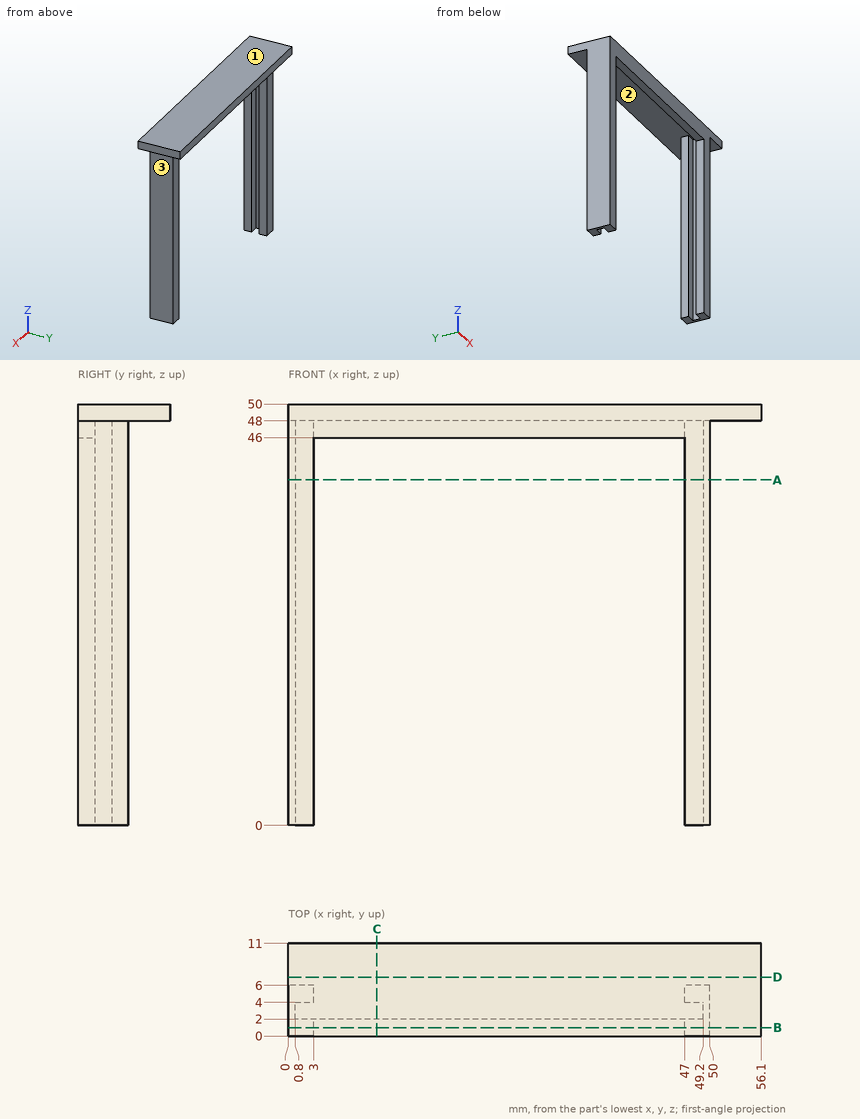
Design review of the part shown in the three views and the two pictorial views. Dimensions are in mm from the part's minimum x, y and z. Round coordinates to 2 decimals unless told otherwise and drop trailing zeros. Loops run counter-clockwise (first coordinate to the right, second up) from the corner with the lowest first, then second, coordinate; pieces in that order, holes last. Notation, with made-up numbers: (60.25, -15) -> (81.25, -15) arc R20 ccw to (81.25, -8) -> close; hole circle Ø10 at (-5.75, -15.75). An arc over 180 degrees is marked (long way). Use one line per item in the form item = value. Start each with the question number.
Q1. We need section D-D on y = 7. Give the boundary of the cut face in (x, z), then the cut area to 3 significant figures.
Q2. We need section B-B on y = 1. Give the boundary of the cut face in (x, z).
Q3. We need section C-C on x = 10.5. Give the boundary of the cut face in (y, z), then the cut area to 3 significant figures.
Q4. We need section A-A on z = 41. Give the boundary of the cut face in (x, y), then the cut area to 3 significant figures.
Q5. Wall thickness on line 1 along X through (y, z) = (5.75, 16); line 2 along X through (y, z) = (3.75, 39); line 3 along Z through (x, y) = (30, 10.25): over which ranges is each line inside the solid? List them lowest first. Write a range as [from, to].
Q6. For pin 1 Ø1 at (y, z) = (4.5, 23.5) entering from -X; pin 2 Ø14.5 at (x, z) = (14, 25.5) entering from +Y; pin 3 Ø0.9 at (x, z) = (48.5, 19) entering from +Y; pin 4 Ø2 at (x, y) = (39, 7) entering from -Z, all flat-tipped, find the tip position at first contact; note any pin that passes through.
Q7. Draft analysis for pull direction X (two halves, no side actions). For the marked faces 1, 2 and 3, state which applies: +X half, -X half, draft (parallel to the pull), parting line (faces both ways), or undercut.
Calculated:
q1.outline = (0, 48) -> (56.1, 48) -> (56.1, 50) -> (0, 50) -> close
q1.area = 112 mm²
q2.outline = (0, 0) -> (3, 0) -> (3, 46) -> (47, 46) -> (47, 0) -> (50, 0) -> (50, 48) -> (56.1, 48) -> (56.1, 50) -> (0, 50) -> close
q3.outline = (0, 46) -> (2, 46) -> (2, 48) -> (11, 48) -> (11, 50) -> (0, 50) -> close
q3.area = 26.0 mm²
q4.outline = (0, 0) -> (3, 0) -> (3, 2) -> (0.8, 2) -> (0.8, 4) -> (3, 4) -> (3, 6) -> (0, 6) -> close; (47, 0) -> (50, 0) -> (50, 6) -> (47, 6) -> (47, 4) -> (49.2, 4) -> (49.2, 2) -> (47, 2) -> close
q4.area = 27.2 mm²
q5.line_1 = [0, 3], [47, 50]
q5.line_2 = [0, 0.8], [49.2, 50]
q5.line_3 = [48, 50]
q6.pin_1 = 0
q6.pin_2 = through
q6.pin_3 = 6
q6.pin_4 = 48
q7.face_1 = draft
q7.face_2 = undercut
q7.face_3 = +X half
